```python
from build123d import *

# Parameters (mm, degrees)
SKETCH1_W                = 203.2
SKETCH1_H                = 152.4
SKETCH1_R                = 25.4
BOSS_EXTRUDE1_DEPTH      = 2.54
BOSS_EXTRUDE2_DEPTH      = 25.4
BOSS_EXTRUDE2_DEPTH_BACK = 27.94
SKETCH2_R                = 27.94
SKETCH2_R_2              = 25.4
CUT_EXTRUDE1_START       = -5.08
SKETCH3_R                = 27.94
SKETCH3_R_2              = 26.67
CUT_EXTRUDE1_DEPTH       = 6.35
SKETCH4_R                = 1.5875
CUT_EXTRUDE2_DEPTH       = 131.037085479
SKETCH5_W                = 203.2
SKETCH5_H                = 2.54
CUT_EXTRUDE3_DEPTH       = 131.037085479


with BuildPart() as part:
    # Sketch1 → Boss-Extrude1 (new body)
    with BuildSketch(Plane(origin=(0, 0, 0), x_dir=(0, 0, -1), z_dir=(1, 0, 0))):
        Rectangle(SKETCH1_W, SKETCH1_H)
        with Locations((50.8, 0)):
            Circle(SKETCH1_R, mode=Mode.SUBTRACT)
        with Locations((-50.8, 0)):
            Circle(SKETCH1_R, mode=Mode.SUBTRACT)
    extrude(amount=BOSS_EXTRUDE1_DEPTH)

    # Sketch2 → Boss-Extrude2 (add, two sides: drawn at the far end of the back side and taken through both)
    # profile 1 of 2: a face of its own
    with BuildSketch(Plane(origin=(2.54, 0, 0), x_dir=(0, 0, -1), z_dir=(1, 0, 0)).offset(-BOSS_EXTRUDE2_DEPTH_BACK)):
        with Locations((-50.8, 0)):
            Circle(SKETCH2_R)
        with Locations((-50.8, 0)):
            Circle(SKETCH2_R_2, mode=Mode.SUBTRACT)
    # profile 2 of 2: a face of its own
    with BuildSketch(Plane(origin=(2.54, 0, 0), x_dir=(0, 0, -1), z_dir=(1, 0, 0)).offset(-BOSS_EXTRUDE2_DEPTH_BACK)):
        with Locations((50.8, 0)):
            Circle(SKETCH2_R)
        with Locations((50.8, 0)):
            Circle(SKETCH2_R_2, mode=Mode.SUBTRACT)
    extrude(amount=BOSS_EXTRUDE2_DEPTH + BOSS_EXTRUDE2_DEPTH_BACK)

    # Sketch3 → Cut-Extrude1 (cut)
    with BuildSketch(Plane(origin=(27.94, 0, 0), x_dir=(0, 0, -1), z_dir=(1, 0, 0)).offset(CUT_EXTRUDE1_START)):
        with Locations((50.8, 0)):
            Circle(SKETCH3_R)
        with Locations((50.8, 0)):
            Circle(SKETCH3_R_2, mode=Mode.SUBTRACT)
    cut_extrude1 = extrude(amount=-CUT_EXTRUDE1_DEPTH, mode=Mode.SUBTRACT)

    # Mirror1: Cut-Extrude1 across plane
    add(cut_extrude1.mirror(Plane.XY), mode=Mode.SUBTRACT)

    # Sketch4 → Cut-Extrude2 (cut, through all)
    with BuildSketch(Plane(origin=(2.54, 0, 0), x_dir=(0, 0, -1), z_dir=(1, 0, 0))):
        with Locations((-88.9, 63.5)):
            Circle(SKETCH4_R)
        with Locations((88.9, 63.5)):
            Circle(SKETCH4_R)
        with Locations((88.9, -63.5)):
            Circle(SKETCH4_R)
        with Locations((-88.9, -63.5)):
            Circle(SKETCH4_R)
    extrude(amount=-CUT_EXTRUDE2_DEPTH, mode=Mode.SUBTRACT)

    # Sketch5 → Cut-Extrude3 (cut, through all)
    with BuildSketch(Plane(origin=(2.54, 0, 0), x_dir=(0, 0, -1), z_dir=(1, 0, 0))):
        with Locations((0, -74.93)):
            Rectangle(SKETCH5_W, SKETCH5_H)
        with Locations((0, 74.93)):
            Rectangle(SKETCH5_W, SKETCH5_H)
    extrude(amount=-CUT_EXTRUDE3_DEPTH, mode=Mode.SUBTRACT)


solid = part.part
```
Design review of the part built by this model. Coordinates are the model's own, in mm. A direction names the side the tool comes from. Give positions to 0.01 mm unless a question says otherwise; leave off trailing zeros. Write each loop counter-clockwise with the first axis right and the second up, starting at its lowest first coordinate (ties: lowest second). Pieces come first, ordered by that corner, then holes.
(1) Add section A-A (z = 50.8). Give the boundary of the cut face in (x, y), and give its area (3 significant figures).
Checked values:
outline: (-25.4, -27.94) - (0, -27.94) - (0, -73.66) - (2.54, -73.66) - (2.54, -27.94) - (16.51, -27.94) - (16.51, -26.67) - (22.86, -26.67) - (22.86, -27.94) - (27.94, -27.94) - (27.94, -25.4) - (-25.4, -25.4) - close; (-25.4, 25.4) - (27.94, 25.4) - (27.94, 27.94) - (22.86, 27.94) - (22.86, 26.67) - (16.51, 26.67) - (16.51, 27.94) - (2.54, 27.94) - (2.54, 73.66) - (0, 73.66) - (0, 27.94) - (-25.4, 27.94) - close
area: 487 mm2
(2) Clearance check with flat-ended pins moving along their axes: pin 1 Ø1.5 at (x, y) = (-1, -30.5) entering from +Z; pin 2 Ø4 at (x, z) = (16, 36) entering from -Y; pin 3 Ø10 at (x, z) = (-13, 78) entering from +Y; pin 4 Ø12 at (x, y) = (-14.5, -27) entering from +Z. State where each tip first meets the part, or that it passes through.
Checked values:
pin 1: passes through
pin 2: stops at y = -24.84
pin 3: stops at y = 16.96
pin 4: stops at z = 69.23
(3) Wall thickness on line 1 along Y through (x, z) = (-5, -50); line 2 along Z through (x, y) = (-2.5, 18.5); line 3 along Z through (x, y) = (-17, -21): over which ranges is each line inside the solid? List them lowest first.
Checked values:
line 1: y = -27.93 to -25.39, 25.39 to 27.93
line 2: z = -71.74 to -68.2, -33.4 to -29.86, 29.86 to 33.4, 68.2 to 71.74
line 3: z = -69.23 to -65.09, -36.51 to -32.37, 32.37 to 36.51, 65.09 to 69.23
(4) Tool access review of faces 1 (the face through (-12.88, 8.39, -77.45)), 2 (the face through (19.73, 8.01, 76.24)), 3 (the face through (25.36, 27.7, 54.44)): name each direction out of +Z, -Z, +X, -X, +Y, -Y from which nothing blocks a thin tool from reaching the whole face with its end or side.
Checked values:
face 1: -X
face 2: none
face 3: +X
(5) Add section B-B (x = -3.5). Give the boundary of the cut face in (y, z).
Checked values:
outline: circle Ø55.88 at (0, -50.8); circle Ø55.88 at (0, 50.8); hole circle Ø50.8 at (0, -50.8); hole circle Ø50.8 at (0, 50.8)
(6) Mouldability with a two-part tool opening along Z and no side actions: class faces 4 (the face through (-12.88, 27.7, 54.44)), 5 (the face through (9.43, 8.39, -77.45)), 6 (the face through (27.94, -25, 45)) as +Z half, -Z half, draft (parallel to the pull), parting line (faces both ways), or undercut.
Checked values:
face 4: undercut
face 5: undercut
face 6: draft
(7) Add section D-D (z = -69.5). Give the boundary of the cut face in (x, y).
Checked values:
outline: (-25.4, -20.76) - (0, -20.76) - (0, -73.66) - (2.54, -73.66) - (2.54, -20.76) - (16.51, -20.76) - (16.51, -19.02) - (22.86, -19.02) - (22.86, -20.76) - (27.94, -20.76) - (27.94, -17.19) - (-25.4, -17.19) - close; (-25.4, 17.19) - (27.94, 17.19) - (27.94, 20.76) - (22.86, 20.76) - (22.86, 19.02) - (16.51, 19.02) - (16.51, 20.76) - (2.54, 20.76) - (2.54, 73.66) - (0, 73.66) - (0, 20.76) - (-25.4, 20.76) - close
(8) Add section C-C (y = 0). Give the number of separate pieces and of enclosed holes in the cut face, and give its area (3 significant figures).
Checked values:
separate pieces: 3
enclosed holes: 0
area: 742 mm2
